```python
from build123d import *

# Parameters (mm, degrees)
EXTRUDE_1_DEPTH     = 5
EXTRUDE_3_DEPTH     = 15
SKETCH_9_W          = 119.641605024
SKETCH_9_H          = 10.286902638
CUT_EXTRUDE_2_DEPTH = 165.924225025
SKETCH_10_R         = 1.982942862
CUT_EXTRUDE_3_DEPTH = 135.907375632
EXTRUDE_5_DEPTH     = 70
SKETCH_14_R         = 28
CUT_EXTRUDE_5_DEPTH = 4.5


with BuildPart() as part:
    # 草图1 → 凸台-拉伸1 (new body)
    with BuildSketch(Plane(origin=(0, 0, 0), x_dir=(1, 0, 0), z_dir=(0, 1, 0))):
        with BuildLine():
            Line((-25, 65), (25, 65))
            ThreePointArc((25, 65), (32.071067812, 62.071067812), (35, 55))
            Line((35, 55), (35, -65))
            Line((35, -65), (-35, -65))
            Line((-35, -65), (-35, 55))
            ThreePointArc((-35, 55), (-32.071067812, 62.071067812), (-25, 65))
        make_face()
    extrude(amount=EXTRUDE_1_DEPTH)

    # 草图8 → 凸台-拉伸3 (add)
    with BuildSketch(Plane(origin=(0, 24.395825623, 42.254809472), x_dir=(1, 0, 0), z_dir=(0, 0.499999999999998, 0.8660254037844398))):
        with BuildLine():
            ThreePointArc((25, 81.830127019), (32.071067812, 78.901194831), (35, 71.830127019))
            Line((35, 71.830127019), (35, -28.169872981))
            Line((35, -28.169872981), (-35, -28.169872981))
            Line((-35, -28.169872981), (-35, 71.830127019))
            ThreePointArc((-35, 71.830127019), (-32.071067812, 78.901194831), (-25, 81.830127019))
            Line((-25, 81.830127019), (25, 81.830127019))
        make_face()
    extrude(amount=-EXTRUDE_3_DEPTH)

    # 草图9 → 切除-拉伸2 (cut, through all)
    with BuildSketch(Plane.XY.offset(65)):
        with Locations((24.820802512, -5.143451319)):
            Rectangle(SKETCH_9_W, SKETCH_9_H)
    extrude(amount=-CUT_EXTRUDE_2_DEPTH, mode=Mode.SUBTRACT)

    # 草图10 → 切除-拉伸3 (cut, through all)
    with BuildSketch(Plane.ZY.offset(35)):
        with Locations((55.11669843, 6.123569619)):
            Circle(SKETCH_10_R)
    extrude(amount=-CUT_EXTRUDE_3_DEPTH, mode=Mode.SUBTRACT)

    # 草图13 → 凸台-拉伸5 (add)
    with BuildSketch(Plane(origin=(35, 0, 0), x_dir=(0, 0, -1), z_dir=(1, 0, 0))):
        with BuildLine():
            Line((-31.802359522, 12.5), (-36.132486541, 5))
            Line((-36.132486541, 5), (-27.472232503, 5))
            ThreePointArc((-27.472232503, 5), (-31.802359522, 7.5), (-31.802359522, 12.5))
        make_face()
    extrude(amount=-EXTRUDE_5_DEPTH)

    # 草图14 → 切除-拉伸5 (cut)
    with BuildSketch(Plane(origin=(0, 24.395825623, 42.254809472), x_dir=(1, 0, 0), z_dir=(0, 0.49999999999999806, 0.8660254037844398))):
        with Locations(Location((0, 41.66372629, 0), (0, 0, 270))):
            Circle(SKETCH_14_R)
    extrude(amount=-CUT_EXTRUDE_5_DEPTH, mode=Mode.SUBTRACT)


solid = part.part
```
For this review, take the finished solid that the model builds, in its own axes (mm). A direction names the side the tool comes from. Round coordinates to 2 decimals unless told otherwise and drop trailing zeros. Write each loop counter-clockwise with the first axis right and the second up, starting at its lowest first coordinate (ties: lowest second). Pieces come first, ordered by that corner, then holes. Notation, with made-up numbers: (60.25, 22) -> (94.25, 22) arc R15 cw to (94.25, 50) -> close; hole circle Ø4 at (26.25, -31.5). An arc over 180 degrees is marked (long way). Use one line per item in the form item = value.
Q1. Consider section C-C (y = 10). State the section outline as (x, z) points.
Resolved:
outline = (-35, 32.47) -> (35, 32.47) -> (35, 50.57) -> (-35, 50.57) -> close
Q2. Clearance check with flat-ended pins moving along their axes: pin 1 Ø8 at (x, y) = (-21.5, 72) entering from -Z; pin 2 Ø6 at (x, y) = (6, 69) entering from -Z; pin 3 Ø2.5 at (x, z) = (9, 60.5) entering from +Y. State where each tip first meets the part, or that it passes through.
Resolved:
pin_1 = -4.86
pin_2 = -2.55
pin_3 = 5
Q3. Consider section B-B (z = -43). State the section outline as (x, y) points, then the cut area to 3 significant figures.
Resolved:
outline = (-35, 0) -> (35, 0) -> (35, 5) -> (-35, 5) -> close
area = 350 mm²
Q4. The part is to be moulded in two halves that separate along Z. For faces 4 (the cylindrical face through (-32.15, 2.46, -61.99)), 5 (the flat face through (0, 2, 65)), 6 (the cylindrical face through (-0.49, 4.14, 55.09)), say which applies: released by +Z, released by -Z, zero draft, split by the parting line, or undercut.
Resolved:
face_4 = released by -Z
face_5 = released by +Z
face_6 = undercut
Q5. Machinability: for faces 1 (the flat face through (0, 5, 61)), 2 (the flat face through (-0.35, 91.57, -5.06)), 3 (the flat face through (0.49, 50.66, 9.77)), which of the approach directions +Z, -Z, +X, -X, +Y, -Y give a long, thin tool a straight path to every point of the face, cutting with its end or side? Answer none if there is none.
Resolved:
face_1 = +Z, +X, -X, +Y
face_2 = -Z, +X, -X, +Y
face_3 = -Z, +X, -X
Q6. To check wall thickness, follow probe 1 along Y at (x, z) = (-21.5, -53); probe 2 along Y at (x, z) = (24, 6); probe 3 along Y at (x, z) = (-10.5, 13). State the ranges of each line that lie inside material, in increasing order. Write a range as from..to.
Resolved:
probe_1 = 0..5
probe_2 = 0..5, 57.19..87.19
probe_3 = 0..5, 45.07..66.07
